Geometry: final body of the model. Coordinates: model frame, mm. A direction names the side the tool comes from. Round coordinates to 2 decimals unless told otherwise and drop trailing zeros. Order: outer loops, then holes, each group sorted by start corner. A loop starts at its lowest first (then second) coordinate and runs counter-clockwise, first axis right, second up. Notation, with made-up numbers: M 15,9 L 67,9 A22 ccw 67,39 Z; hole C 22,12.25 d6. An arc over 180 degrees is marked long. Put each result on its own line as item: value. Start each with the question number.
1) Section A-A, the plane x = 0. Return loops of the section in (y, z).
2) Section B-B, the plane z = 0. Return loops of the section in (x, y).
3) Section C-C, the plane y = -2.95. Return loops of the section in (x, z).
4) Section D-D, the plane x = -8.5. Return loops of the section in (y, z), then the cut area to 3 significant figures.
5) Access query for faces 1 (the flat face through (9.5, -2, 13)), 2 (the flat face through (-10.093, -2, 13)), 3 (the flat face through (-10.5, -2, -2)), 4 (the flat face through (0, -2, -12.872)). Directions: +Z, -Z, +X, -X, +Y, -Y. A direction counts if a zero-diameter tool reaches every point of the face in a straight line with its end or side. Return the directions, or none.
6) Material intervals for probe 1 along Z at (x, y) = (0, -0.9); probe 2 along Z at (x, y) = (2, -2.85); probe 3 along X at (y, z) = (-1.25, -7), sorted ascending. Write a range as [from, to].
7) First-contact query: P1, Ø1.8, axis at y = -2.5, z = 13.5, coming from the +X side; P2, Ø2, axis at x = 0.5, z = -10.5, coming from the +Y side; P3, Ø1, axis at x = 6.5, y = -1.5, coming from the +Z side; P4, Ø1.8, axis at y = -1.5, z = 13.5, coming from the -X side. Flat tips, straight axial feed; report the tip coordinate or a pass-through.
8) Draft query along Z for faces 5 (the flat face through (10.093, -2, 13)), 6 (the flat face through (0, -2, 10.662)), 7 (the cylindrical face through (5.616, -1.726, -14.361)), 8 (the cylindrical face through (-1.73, -1.73, -7.81)). Return one class per face: pulls with the +Z half, pulls with the -Z half, needs draft (parallel to the pull), parting line crosses it, or undercut.
from build123d import *

# Parameters (mm, degrees)
F0_R        = 8
F1_DEPTH    = 3.5
F2_T4_DEPTH = 14.2095720734
F2_T9_DEPTH = 14.2095720734


# Not quite as in the source:
# - a fillet or chamfer that OpenCascade refuses, or shapes differently, is made with other operations: its cross-section is extruded or revolved along the edge and cut away or added


with BuildPart() as f1:
    # F0 (on Front) → F1 (new body)
    with BuildSketch(Plane.XZ):
        Polygon((5, -15), (10.5, -15), (10.5, 11.1734773964), (10.0929150358, 11.1734773964), (10.0929150358, 15), (9.5, 15), (9.5, 10.6615237892), (-9.5, 10.6615237892), (-9.5, 15), (-10.0929150358, 15), (-10.0929150358, 11.1734773964), (-10.5, 11.1734773964), (-10.5, -15), (-5, -15), (-5, -12.8721727654), (5, -12.8721727654), align=None)
        Circle(F0_R, mode=Mode.SUBTRACT)
    extrude(amount=F1_DEPTH)

    # F2: fillet of radius 2.1419144147 on 2 edges, made by hand


with BuildPart() as f2_tool2:
    # F2_s3 → F2_t4 (new body)
    with BuildSketch(Plane.XZ.offset(-5.3547860367)):
        with BuildLine():
            ThreePointArc((-7.1419144147, -15), (-5.6273522073, -14.3726477927), (-5, -12.8580855853))
            Line((-5, -12.8580855853), (-5, -15))
            Line((-5, -15), (-7.1419144147, -15))
        make_face()
    extrude(amount=F2_T4_DEPTH)

    split(bisect_by=Plane.XY.offset(-12.8721727654), keep=Keep.BOTTOM)


with BuildPart() as f1_1:
    add(f1.part)

    # F2_t1: cut F2_tool2
    add(f2_tool2.part, mode=Mode.SUBTRACT)


with BuildPart() as f2_tool7:
    # F2_s8 → F2_t9 (new body)
    with BuildSketch(Plane.XZ.offset(-5.3547860367)):
        with BuildLine():
            ThreePointArc((5, -12.8580855853), (5.6273522073, -14.3726477927), (7.1419144147, -15))
            Line((7.1419144147, -15), (5, -15))
            Line((5, -15), (5, -12.8580855853))
        make_face()
    extrude(amount=F2_T9_DEPTH)

    split(bisect_by=Plane.XY.offset(-12.8721727654), keep=Keep.BOTTOM)


with BuildPart() as f1_2:
    add(f1_1.part)

    # F2_t6: cut F2_tool7
    add(f2_tool7.part, mode=Mode.SUBTRACT)


solid = f1_2.part
Result sheet:
1. outline: M -3.5,-12.87 L 0,-12.87 L 0,-8 L -3.5,-8 Z; M -3.5,8 L 0,8 L 0,10.66 L -3.5,10.66 Z
2. outline: M -10.5,-3.5 L -8,-3.5 L -8,0 L -10.5,0 Z; M 8,-3.5 L 10.5,-3.5 L 10.5,0 L 8,0 Z
3. outline: M -10.5,-15 L -7.14,-15 A2.14 ccw -5,-12.87 L 5,-12.87 A2.14 ccw 7.14,-15 L 10.5,-15 L 10.5,11.17 L 10.09,11.17 L 10.09,15 L 9.5,15 L 9.5,10.66 L -9.5,10.66 L -9.5,15 L -10.09,15 L -10.09,11.17 L -10.5,11.17 Z; hole C 0,0 d16
4. outline: M -3.5,-15 L 0,-15 L 0,10.66 L -3.5,10.66 Z
4. area: 89.8 mm2
5. face 1: +Z, +Y, -Y
5. face 2: +Z, -X, +Y, -Y
5. face 3: +Z, -Z, -X, +Y, -Y
5. face 4: -Z, +Y, -Y
6. probe 1: z = [-12.87, -8], [8, 10.66]
6. probe 2: z = [-12.87, -7.75], [7.75, 10.66]
6. probe 3: x = [-10.5, -3.87], [3.87, 10.5]
7. P1: stops at x = 10.09
7. P2: stops at y = 0
7. P3: stops at z = 10.66
7. P4: stops at x = -10.09
8. face 5: needs draft
8. face 6: pulls with the +Z half
8. face 7: pulls with the -Z half
8. face 8: undercut
